Input: part model. Units: mm. Frame: model coordinates. Face numbers are marked on the shaded views. Round coordinates to 2 decimals unless told otherwise and drop trailing zeros. Loops run counter-clockwise (first coordinate to the right, second up) from the corner with the lowest first, then second, coordinate; pieces in that order, holes last.
(1) Line query: line 1 (Z direction, x = 0, y = 4.4); line 2 (Y direction, x = -1, z = 75.5); line 3 (Z direction, x = 4.75, y = 0). Output: solid intervals per line, ascending.
(2) Draft query along Y for the marked faces 1, 2, 3 and 4. Return one class per face: released by +Y, released by -Y, zero draft, split by the parting line, or undercut.
(3) Cut plane A-A, the plane x = -2.5. Output: boundary loops of the cut face in (y, z).
(4) Cut plane B-B, the plane y = 0. Give the number of separate pieces and of enclosed holes in the cut face, and give its area (3 significant figures).
(5) Cut plane C-C, the plane z = 24.5. Output: boundary loops of the cut face in (x, y).
(6) Cut plane D-D, the plane z = 56. Output: boundary loops of the cut face in (x, y).
(7) First-contact query: pin 1 Ø4 at (x, z) = (0, 5) entering from +Y. Flat tip, straight axial feed; report the tip coordinate or a pass-through.
from build123d import *

# Parameters (mm, degrees)
SKETCH_1_W          = 10
SKETCH_1_H          = 10
SKETCH_1_W_2        = 8
SKETCH_1_H_2        = 8
EXTRUDE_1_DEPTH     = 80
SKETCH_2_R          = 1.6
CUT_EXTRUDE_1_DEPTH = 81.777472107
SKETCH_3_R          = 1.6
CUT_EXTRUDE_2_DEPTH = 81.777472107
SKETCH_4_R          = 1.6
CUT_EXTRUDE_3_DEPTH = 81.777472107
SKETCH_5_R          = 1.6
CUT_EXTRUDE_4_DEPTH = 81.777472107
SKETCH_6_R          = 1.6
CUT_EXTRUDE_5_DEPTH = 81.777472107
SKETCH_7_R          = 2.15
CUT_EXTRUDE_6_DEPTH = 81.777472107


with BuildPart() as part:
    # ｽｹｯﾁ1 → 押し出し-薄板1 (new body)
    with BuildSketch(Plane.XY):
        Rectangle(SKETCH_1_W, SKETCH_1_H)
        Rectangle(SKETCH_1_W_2, SKETCH_1_H_2, mode=Mode.SUBTRACT)
    extrude(amount=EXTRUDE_1_DEPTH)

    # ｽｹｯﾁ2 → ｶｯﾄ - 押し出し1 (cut, through all)
    with BuildSketch(Plane(origin=(0, 5, 0), x_dir=(1, 0, 0), z_dir=(0, 1, 0))):
        with Locations(Location((0, -5, 0), (0, 0, 180))):
            Circle(SKETCH_2_R)
    extrude(amount=-CUT_EXTRUDE_1_DEPTH, mode=Mode.SUBTRACT)

    # ｽｹｯﾁ3 → ｶｯﾄ - 押し出し2 (cut, through all)
    with BuildSketch(Plane(origin=(5, 0, 0), x_dir=(0, 0, -1), z_dir=(1, 0, 0))):
        with Locations(Location((-15, 0, 0), (0, 0, 90))):
            Circle(SKETCH_3_R)
    extrude(amount=-CUT_EXTRUDE_2_DEPTH, mode=Mode.SUBTRACT)

    # ｽｹｯﾁ4 → ｶｯﾄ - 押し出し3 (cut, through all)
    with BuildSketch(Plane.XZ.offset(5)):
        with Locations((0, 65)):
            Circle(SKETCH_4_R)
        with Locations((0, 56)):
            Circle(SKETCH_4_R)
    extrude(amount=-CUT_EXTRUDE_3_DEPTH, mode=Mode.SUBTRACT)

    # ｽｹｯﾁ5 → ｶｯﾄ - 押し出し4 (cut, through all)
    with BuildSketch(Plane.ZY.offset(5)):
        with Locations(Location((50, 0, 0), (0, 0, 270))):
            Circle(SKETCH_5_R)
    extrude(amount=-CUT_EXTRUDE_4_DEPTH, mode=Mode.SUBTRACT)

    # ｽｹｯﾁ6 → ｶｯﾄ - 押し出し5 (cut, through all)
    with BuildSketch(Plane(origin=(0, 5, 0), x_dir=(1, 0, 0), z_dir=(0, 1, 0))):
        with Locations(Location((0, -43, 0), (0, 0, 180))):
            Circle(SKETCH_6_R)
        with Locations(Location((0, -28, 0), (0, 0, 180))):
            Circle(SKETCH_6_R)
    extrude(amount=-CUT_EXTRUDE_5_DEPTH, mode=Mode.SUBTRACT)

    # ｽｹｯﾁ7 → ｶｯﾄ - 押し出し6 (cut, through all)
    with BuildSketch(Plane(origin=(5, 0, 0), x_dir=(0, 0, -1), z_dir=(1, 0, 0))):
        with Locations(Location((-75, 0, 0), (0, 0, 90))):
            Circle(SKETCH_7_R)
    extrude(amount=-CUT_EXTRUDE_6_DEPTH, mode=Mode.SUBTRACT)


solid = part.part
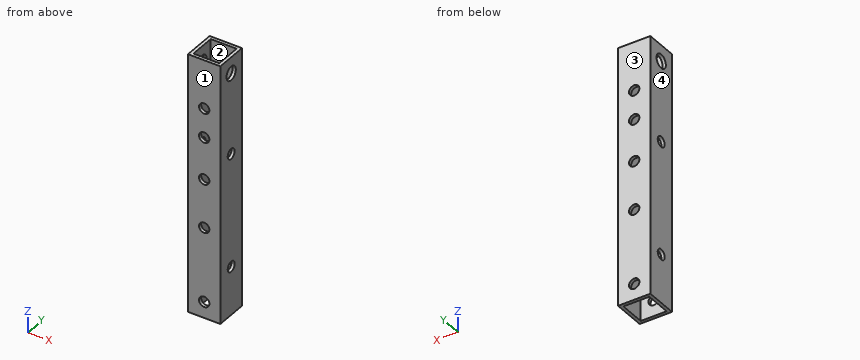
Reported:
1. line 1: z = 0 to 3.4, 6.6 to 26.4, 29.6 to 41.4, 44.6 to 54.4, 57.6 to 63.4, 66.6 to 80
1. line 2: y = -5 to -4, 4 to 5
1. line 3: z = 0 to 13.4, 16.6 to 48.4, 51.6 to 72.85, 77.15 to 80
2. face 1: released by -Y
2. face 2: undercut
2. face 3: released by +Y
2. face 4: zero draft
3. outline: (-5, 0) - (-4, 0) - (-4, 80) - (-5, 80) - close; (4, 0) - (5, 0) - (5, 80) - (4, 80) - close
4. separate pieces: 8
4. enclosed holes: 0
4. area: 139 mm2
5. outline: (-5, -5) - (5, -5) - (5, 5) - (-5, 5) - close; hole (-4, -4) - (4, -4) - (4, 4) - (-4, 4) - close
6. outline: (-5, -5) - (-1.6, -5) - (-1.6, -4) - (-4, -4) - (-4, 4) - (-1.6, 4) - (-1.6, 5) - (-5, 5) - close; (1.6, -5) - (5, -5) - (5, 5) - (1.6, 5) - (1.6, 4) - (4, 4) - (4, -4) - (1.6, -4) - close
7. pin 1: stops at y = 5
